from build123d import *

# Parameters (mm, degrees)
F0_W     = 10
F0_H     = 10
F0_W_2   = 30
F1_DEPTH = 30


with BuildPart() as f1:
    # F0 (on Front) → F1 (new body)
    with BuildSketch(Plane.XZ):
        with Locations((-55, 25)):
            Rectangle(F0_W, F0_H)
        with BuildLine():
            Line((15, 0), (7.5, 0))
            ThreePointArc((7.5, 0), (5.303301, -5.303301), (0, -7.5))
            Line((0, -7.5), (0, -20))
            Line((0, -20), (15, -20))
            Line((15, -20), (15, 0))
        make_face()
        with BuildLine():
            ThreePointArc((0, -7.5), (-5.303301, 5.303301), (7.5, 0))
            Line((7.5, 0), (15, 0))
            Line((15, 0), (15, 30))
            Line((15, 30), (-50, 30))
            Line((-50, 30), (-50, 20))
            Line((-50, 20), (-60, 20))
            Line((-60, 20), (-60, -20))
            Line((-60, -20), (0, -20))
            Line((0, -20), (0, -7.5))
        make_face()
        with Locations((-35, 15)):
            Rectangle(F0_W_2, F0_H, mode=Mode.SUBTRACT)
    extrude(amount=F1_DEPTH)


solid = f1.part
The model under review builds one solid part; all positions refer to its coordinate system, in mm. A direction names the side the tool comes from. Round coordinates to 2 decimals unless told otherwise and drop trailing zeros. Loops run counter-clockwise (first coordinate to the right, second up) from the corner with the lowest first, then second, coordinate; pieces in that order, holes last. Notation, with made-up numbers: (-14, -25) -> (34, -25) arc R36 ccw to (34, 9) -> close; hole circle Ø2 at (51, 66.5). An arc over 180 degrees is marked (long way). One line per question, with ' | ' between items. Start each with the question number.
Item 1: For pin 1 (13.5 mm diameter, centred on x = 0, z = 0, fed in from +Y) (3 decimals), flat-tipped, find the tip position at first contact; note if it passes through.
Item 2: Add section C-C, the plane y = -15.5. Write out the cut boundary in (x, z).
Item 3: Draft analysis for pull direction Z (two halves, no side actions). For faces 3 (the face through (-23, -30, 5)), 4 (the face through (-35, -15, 20)), 5 (the face through (-23, -15, -20)), state which applies: +Z half, -Z half, draft (parallel to the pull), parting line (faces both ways), or undercut.
Item 4: Wall thickness on line 1 along Z through (x, y) = (0, -14.75); line 2 along X through (y, z) = (-14.75, 0); line 3 along Z through (x, y) = (-33.5, -19.5): over which ranges is each line inside the solid? List them lowest first. Write a range as [from, to].
Item 5: Machinability: for faces 1 (the face through (-20, -15, 15)), 2 (the face through (-23, 0, 5)), which of the approach directions +Z, -Z, +X, -X, +Y, -Y give a long, thin tool a straight path to every point of the face, cutting with its end or side? Answer none if there is none.
Item 6: Add section A-A, the plane z = 13. Write out the cut boundary in (x, y), then the cut area to 3 significant figures.
Item 7: Add section B-B, the plane x = -1. Write out the cut boundary in (y, z), then the cut area to 3 significant figures.
Return value:
1) pin 1: passes through
2) outline: (-60, -20) -> (15, -20) -> (15, 30) -> (-60, 30) -> close; hole (-50, 10) -> (-20, 10) -> (-20, 20) -> (-50, 20) -> close; hole circle Ø15 at (0, 0)
3) face 3: draft | face 4: undercut | face 5: -Z half
4) line 1: z = [-20, -7.5], [7.5, 30] | line 2: x = [-60, -7.5], [7.5, 15] | line 3: z = [-20, 10], [20, 30]
5) face 1: +Y, -Y | face 2: +Z, -Z, +X, -X, +Y
6) outline: (-60, -30) -> (-50, -30) -> (-50, 0) -> (-60, 0) -> close; (-20, -30) -> (15, -30) -> (15, 0) -> (-20, 0) -> close | area: 1,350 mm2
7) outline: (-30, -20) -> (0, -20) -> (0, -7.43) -> (-30, -7.43) -> close; (-30, 7.43) -> (0, 7.43) -> (0, 30) -> (-30, 30) -> close | area: 1,050 mm2
